Model file for the job. Use its own axes, mm. A direction names the side the tool comes from. Give positions to 0.01 mm unless a question says otherwise; leave off trailing zeros. Write each loop counter-clockwise with the first axis right and the second up, starting at its lowest first coordinate (ties: lowest second). Pieces come first, ordered by that corner, then holes.
```python
from build123d import *

# Parameters (mm, degrees)
EXTRUDE_1_DEPTH    = 10
HOLE_WIZARD_M3_1_D = 2.5
SKETCH_6_R         = 4
EXTRUDE_2_DEPTH    = 15


with BuildPart() as part:
    # 草图2 → 凸台-拉伸1 (new body)
    with BuildSketch(Plane(origin=(0, 0, 0), x_dir=(1, 0, 0), z_dir=(0, 1, 0))):
        Polygon((37.5, 7.5), (30.587879709, 7.5), (30.587879709, 17), (22.587879709, 17), (22.587879709, 7.5), (-12.412120291, 7.5), (-12.412120291, 13), (-20.412120291, 13), (-20.412120291, 7.5), (-37.5, 7.5), (-37.5, -7.5), (-20.412120291, -7.5), (-20.412120291, -13), (-12.412120291, -13), (-12.412120291, -7.5), (22.587879709, -7.5), (22.587879709, -17), (30.587879709, -17), (30.587879709, -7.5), (37.5, -7.5), align=None)
    extrude(amount=EXTRUDE_1_DEPTH)

    # M3 螺纹孔1 (through all)
    with Locations(Plane(origin=(0, 10, 0), x_dir=(1, 0, 0), z_dir=(0, 1, 0))):
        with Locations((-16.412120291, 10), (-16.412120291, -10), (26.587879709, 14), (26.587879709, -14)):
            Hole(HOLE_WIZARD_M3_1_D / 2)

    # 草图6 → 凸台-拉伸2 (add)
    with BuildSketch(Plane.XY.offset(7.5)):
        with BuildLine():
            Line((-37.5, 0), (37.5, 0))
            Line((37.5, 0), (37.5, -9.298476379))
            ThreePointArc((37.5, -9.298476379), (25.5, -21.298476379), (13.5, -9.298476379))
            Line((13.5, -9.298476379), (-28.201523621, -9.298476379))
            Line((-28.201523621, -9.298476379), (-37.5, 0))
        make_face()
        with Locations((25.5, -9.298476379)):
            Circle(SKETCH_6_R, mode=Mode.SUBTRACT)
    extrude(amount=-EXTRUDE_2_DEPTH)


solid = part.part
```
1. Slice it at B-B, the plane x = 27. Write the cut outline in (y, z), and give its area (3 significant figures).
Calculated:
outline: (-21.2, -7.5) - (-13.01, -7.5) - (-13.01, 7.5) - (-21.2, 7.5) - close; (-5.59, -7.5) - (0, -7.5) - (0, -12.82) - (10, -12.82) - (10, 12.82) - (0, 12.82) - (0, 7.5) - (-5.59, 7.5) - close; (0, -17) - (10, -17) - (10, -15.18) - (0, -15.18) - close; (0, 15.18) - (10, 15.18) - (10, 17) - (0, 17) - close
area: 500 mm2
2. Which spindle directions (+Z, -Z, +X, -X, +Y, -Y) get a long thin tool onto all of the face, cutting with end or side? Do faces 1 (the flat face through (-20.412, 5, -10)), 2 (the flat face through (30.588, 5, -12)), 3 (the flat face through (-16, 5, 13)), 4 (the flat face through (-16, 0, -12)), 5 (the flat face through (22.588, 5, -12)). Say none if no direction does.
Calculated:
face 1: -Z, -X, +Y, -Y
face 2: -Z, +X, +Y, -Y
face 3: +Z, -X, +Y, -Y
face 4: -Z, +X, -X, -Y
face 5: -Z, +Y, -Y
3. Pull direction Z, two halves, no side cores. Call faces 6 (the cylindrical face through (25.396, 4.93, -14.375)), 7 (the flat face through (-20.412, 5, 10)), 8 (the flat face through (-16, 5, -13)): +Z half, -Z half, draft (parallel to the pull), parting line (faces both ways), or undercut.
Calculated:
face 6: undercut
face 7: draft
face 8: -Z half
4. Pin check, flat tips, straight feed: P1, Ø1.5, axis at y = -10, z = 1.5, coming from the -X side; P2, Ø12, axis at x = 24.5, z = -4.5, coming from the -Y side; P3, Ø3, axis at y = 5.5, z = -13.5, coming from the -X side; P4, Ø3, axis at x = 26.59, z = 14, coming from the -Y side. Stop position of each tip, or through.
Calculated:
P1: stops at x = -28.25
P2: stops at y = -21.3
P3: stops at x = -20.41
P4: stops at y = 0
5. Probe probe 1 along X at (y, z) = (7.5, -10); probe 2 along Z at (x, y) = (-10, -9); probe 3 along Y at (x, z) = (29, -8). List the from-to ranges inside material, lowest first.
Calculated:
probe 1: x = -20.41 to -17.66, -15.16 to -12.41, 22.59 to 30.59
probe 2: z = -7.5 to 7.5
probe 3: y = 0 to 10
6. Slice it at C-C, the plane z = -14. Write the cut outline in (x, y).
Calculated:
outline: (22.59, 0) - (25.34, 0) - (25.34, 10) - (22.59, 10) - close; (27.84, 0) - (30.59, 0) - (30.59, 10) - (27.84, 10) - close
7. Slice it at A-A, the plane z = 10. Write the cut outline in (x, y).
Calculated:
outline: (-20.41, 0) - (-17.66, 0) - (-17.66, 10) - (-20.41, 10) - close; (-15.16, 0) - (-12.41, 0) - (-12.41, 10) - (-15.16, 10) - close; (22.59, 0) - (30.59, 0) - (30.59, 10) - (22.59, 10) - close
8. Slice it at D-D, the plane y = 3. Write the cut outline in (x, z), and give its area (3 significant figures).
Calculated:
outline: (-37.5, -7.5) - (-20.41, -7.5) - (-20.41, -13) - (-12.41, -13) - (-12.41, -7.5) - (22.59, -7.5) - (22.59, -17) - (30.59, -17) - (30.59, -7.5) - (37.5, -7.5) - (37.5, 7.5) - (30.59, 7.5) - (30.59, 17) - (22.59, 17) - (22.59, 7.5) - (-12.41, 7.5) - (-12.41, 13) - (-20.41, 13) - (-20.41, 7.5) - (-37.5, 7.5) - close; hole circle Ø2.5 at (-16.41, -10); hole circle Ø2.5 at (-16.41, 10); hole circle Ø2.5 at (26.59, -14); hole circle Ø2.5 at (26.59, 14)
area: 1,350 mm2
